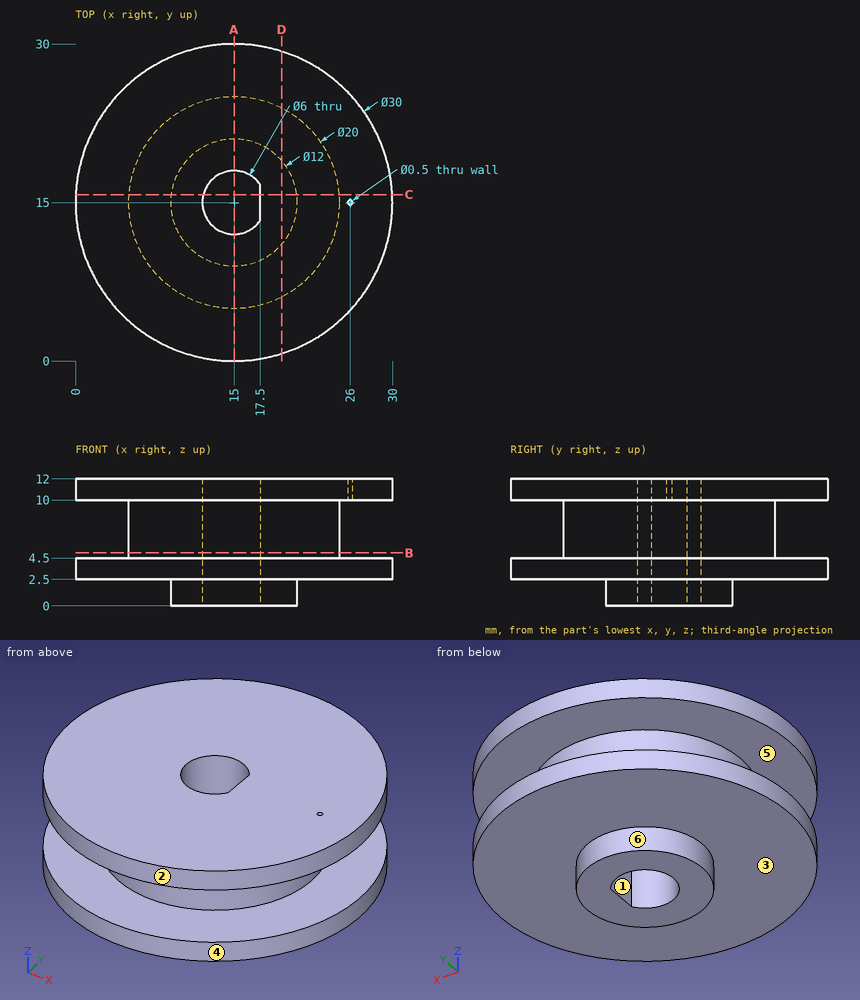
For this review, use the dimensioned drawing (mm, ordinates from the lowest corner) and the shaded views. A direction names the side the tool comes from. Coordinates: 2 decimals unless noted, no trailing zeros. Loops run counter-clockwise (first coordinate to the right, second up) from the corner with the lowest first, then second, coordinate; pieces in that order, holes last. Notation, with made-up numbers: M -30.5,-35.5 L -0.5,-35.5 A24 cw -0.5,-1.5 Z; hole C -3,-19.75 d1. An arc over 180 degrees is marked long. Answer as CSV lines item,"result".
Item 1: Add section A-A on x = 15. State the section outline as (y, z) points.
Answer list:
outline,"M 0,2.5 L 9,2.5 L 9,0 L 12,0 L 12,12 L 0,12 L 0,10 L 5,10 L 5,4.5 L 0,4.5 Z; M 18,0 L 21,0 L 21,2.5 L 30,2.5 L 30,4.5 L 25,4.5 L 25,10 L 30,10 L 30,12 L 18,12 Z"
Item 2: For P1, Ø1.7, axis at y = 14.5, z = 6, coming from the -X side; P2, Ø3, axis at y = 5.5, z = 7, coming from the +X side; P3, Ø6, axis at x = 19.5, z = 6, coming from the -Y side, all flat-tipped, find the tip position at first contact; note any pin that passes through.
Answer list:
P1,"x = 5"
P2,"x = 21"
P3,"y = 0.12"
Item 3: Add section D-D on x = 19.5. State the section outline as (y, z) points, plus the area to 3 significant figures.
Answer list:
outline,"M 0.69,2.5 L 11.03,2.5 L 11.03,0 L 18.97,0 L 18.97,2.5 L 29.31,2.5 L 29.31,4.5 L 23.93,4.5 L 23.93,10 L 29.31,10 L 29.31,12 L 0.69,12 L 0.69,10 L 6.07,10 L 6.07,4.5 L 0.69,4.5 Z"
area,"233 mm²"
Item 4: Add section C-C on y = 15.75. State the section outline as (x, z) points, plus the area to 3 significant figures.
Answer list:
outline,"M 0.02,2.5 L 9.05,2.5 L 9.05,0 L 12.1,0 L 12.1,12 L 0.02,12 L 0.02,10 L 5.03,10 L 5.03,4.5 L 0.02,4.5 Z; M 17.5,0 L 20.95,0 L 20.95,2.5 L 29.98,2.5 L 29.98,4.5 L 24.97,4.5 L 24.97,10 L 29.98,10 L 29.98,12 L 17.5,12 Z"
area,"194 mm²"
Item 5: Machinability: for the marked faces 4, 5 and 6, which of the approach directions +Z, -Z, +X, -X, +Y, -Y give a long, thin tool a straight path to every point of the face, cutting with its end or side? Answer none if there is none.
Answer list:
face 4,"+Z, -Z"
face 5,"none"
face 6,"-Z"
Item 6: For probe 1 along Z at (x, y) = (17, 2.75); probe 2 along Z at (x, y) = (23.5, 12.25); probe 3 along Y at (x, z) = (26, 11), list the stretches that pass through material, from the lowest coordinate up.
Answer list:
probe 1,"2.5 to 4.5, 10 to 12"
probe 2,"2.5 to 12"
probe 3,"4.8 to 14.75, 15.25 to 25.2"
Item 7: Add section B-B on z = 5. State the section outline as (x, y) points, plus the area to 3 significant figures.
Answer list:
outline,"C 15,15 d20; hole M 17.5,13.34 L 17.5,16.66 A3 ccw long Z"
area,"287 mm²"
Item 8: The part is to be moulded in two halves that separate along X. For the marked faces 1, 2 and 3, say which applies: pulls with the +X half, pulls with the -X half, needs draft (parallel to the pull), parting line crosses it, or undercut.
Answer list:
face 1,"undercut"
face 2,"parting line crosses it"
face 3,"needs draft"
